Source: CAD feature listing. Evaluate the final solid. Frame: model axes, mm. Give positions to 0.01 mm unless a question says otherwise; leave off trailing zeros. Loops run counter-clockwise (first coordinate to the right, second up) from the corner with the lowest first, then second, coordinate; pieces in that order, holes last. Notation, with made-up numbers: (-2.5, 14.5) - (3.5, 14.5) arc R17 ccw to (3.5, 22.5) - close; hole circle Ø7 at (88, -21.75). An arc over 180 degrees is marked (long way). Put each result on its own line as item: value.
```python
from build123d import *

# Parameters (mm, degrees)
SKETCH_W  = 480
SKETCH_H  = 40
SKETCH_R  = 8.5
PAD_DEPTH = 20


with BuildPart() as part:
    # Sketch → Pad (new body)
    with BuildSketch(Plane.XZ):
        Rectangle(SKETCH_W, SKETCH_H)
        with Locations((-40, 0)):
            Circle(SKETCH_R, mode=Mode.SUBTRACT)
        with Locations((40, 0)):
            Circle(SKETCH_R, mode=Mode.SUBTRACT)
    extrude(amount=PAD_DEPTH)


solid = part.part
```
1) Section query B-B, the plane z = 4. Output: boundary loops of the cut face in (x, y), plus the area to 3 significant figures.
Check result:
outline: (-240, -20) - (-47.5, -20) - (-47.5, 0) - (-240, 0) - close; (-32.5, -20) - (32.5, -20) - (32.5, 0) - (-32.5, 0) - close; (47.5, -20) - (240, -20) - (240, 0) - (47.5, 0) - close
area: 9,000 mm²
2) Material intervals for line 1 along Z through (x, y) = (40, -5); line 2 along X through (y, z) = (-12, 2.5); line 3 along X through (y, z) = (-14.5, 0.5), sorted ascending. Write a range as [from, to].
Check result:
line 1: [-20, -8.5], [8.5, 20]
line 2: [-240, -48.12], [-31.88, 31.88], [48.12, 240]
line 3: [-240, -48.49], [-31.51, 31.51], [48.49, 240]
3) Mould query, pull axis X, two halves, no side actions, for faces 1 (the flat face through (-3, -10, 20)), 2 (the flat face through (-240, -10, 0)), 3 (the cylindrical face through (-46.265, -9.86, 5.745)). Classes: pulls with the +X half, pulls with the -X half, needs draft (parallel to the pull), parting line crosses it, or undercut.
Check result:
face 1: needs draft
face 2: pulls with the -X half
face 3: undercut
4) Section query C-C, the plane y = -13.5. Output: boundary loops of the cut face in (x, z).
Check result:
outline: (-240, -20) - (240, -20) - (240, 20) - (-240, 20) - close; hole circle Ø17 at (-40, 0); hole circle Ø17 at (40, 0)
5) Section query A-A, the plane x = -40. Output: boundary loops of the cut face in (y, z), plus the area to 3 significant figures.
Check result:
outline: (-20, -20) - (0, -20) - (0, -8.5) - (-20, -8.5) - close; (-20, 8.5) - (0, 8.5) - (0, 20) - (-20, 20) - close
area: 460 mm²
